Could you check a few things on this drawing? It's one solid part, dimensions in mm from its lowest x, y, z. Coordinates: 2 decimals unless noted, no trailing zeros. Order: outer loops, then holes, each group sorted by start corner. A loop starts at its lowest first (then second) coordinate and runs counter-clockwise, first axis right, second up. Notation, with made-up numbers: (22.5, -1) - (37.5, -1) arc R16 cw to (37.5, 19) - close; hole circle Ø3 at (78, 38). An arc over 180 degrees is marked (long way). Answer in a Markdown table with one row per item. Add a question column.
Item 1: I want a section at B-B (x = 12). Please give me the cut outline in (y, z).
Item 2: If I drill on line 1 along Y through (x, z) = (32, 1.3); line 2 along Y through (x, z) = (71, 2.8); line 3 along X through (y, z) = (2.5, 0.85), over which ranges is the centre line in solid material (lowest first)? Write a range as from..to.
Item 3: I want a section at A-A (y = 8). Please give me the cut outline in (x, z), plus the area to 3 significant figures.
Item 4: I want a section at C-C (z = 2.2). Please give me the cut outline in (x, y), plus the area to 3 significant figures.
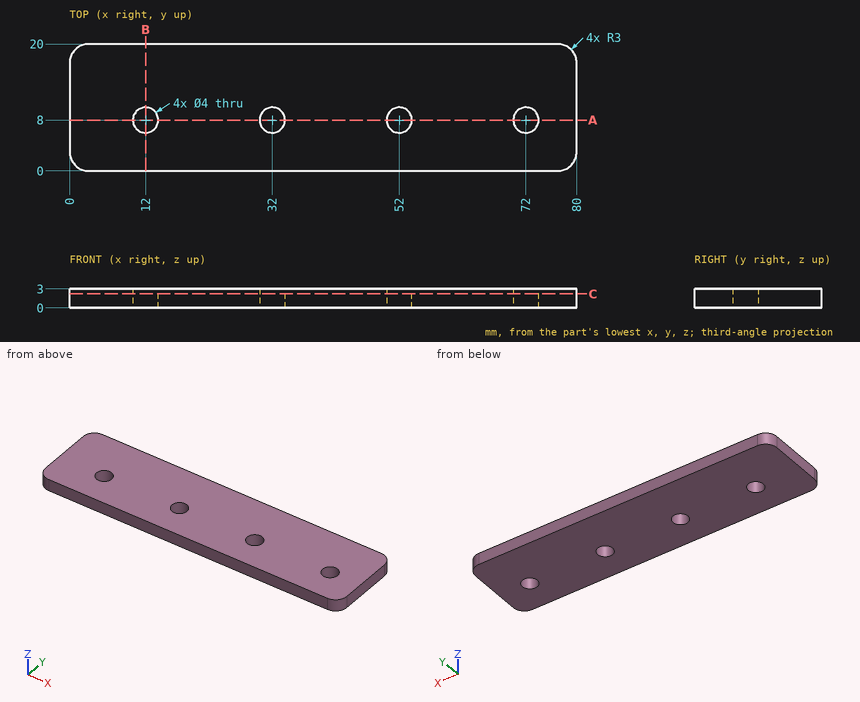
Values follow:
| question | item | result |
|---|---|---|
| 1 | outline | (0, 0) - (6, 0) - (6, 3) - (0, 3) - close; (10, 0) - (20, 0) - (20, 3) - (10, 3) - close |
| 2 | line 1 | y = 0..6, 10..20 |
| 2 | line 2 | y = 0..6.27, 9.73..20 |
| 2 | line 3 | x = 0.04..79.96 |
| 3 | outline | (0, 0) - (10, 0) - (10, 3) - (0, 3) - close; (14, 0) - (30, 0) - (30, 3) - (14, 3) - close; (34, 0) - (50, 0) - (50, 3) - (34, 3) - close; (54, 0) - (70, 0) - (70, 3) - (54, 3) - close; (74, 0) - (80, 0) - (80, 3) - (74, 3) - close |
| 3 | area | 192 mm^2 |
| 4 | outline | (0, 3) arc R3 ccw to (3, 0) - (77, 0) arc R3 ccw to (80, 3) - (80, 17) arc R3 ccw to (77, 20) - (3, 20) arc R3 ccw to (0, 17) - close; hole circle Ø4 at (12, 8); hole circle Ø4 at (32, 8); hole circle Ø4 at (52, 8); hole circle Ø4 at (72, 8) |
| 4 | area | 1,540 mm^2 |
